```python
from build123d import *

# Parameters (mm, degrees)
F1_DEPTH = 20


with BuildPart() as f1:
    # F0 (on Top) → F1 (new body)
    with BuildSketch(Plane.XY):
        with BuildLine():
            Line((-12, 1.6), (-12, 0))
            Line((-12, 0), (0, 0))
            Line((0, 0), (0, 10))
            Line((0, 10), (-18, 10))
            Line((-18, 10), (-18, 8.4))
            ThreePointArc((-18, 8.4), (-10.814003, 7.009238), (-3.505098, 7.4))
            Line((-3.505098, 7.4), (-3.505098, 1.6))
            Line((-3.505098, 1.6), (-12, 1.6))
        make_face()
    extrude(amount=F1_DEPTH)


solid = f1.part
```
Geometry: final body of the model. Coordinates: model frame, mm. A direction names the side the tool comes from. Give positions to 0.01 mm unless a question says otherwise; leave off trailing zeros. Loops run counter-clockwise (first coordinate to the right, second up) from the corner with the lowest first, then second, coordinate; pieces in that order, holes last. Notation, with made-up numbers: (71.5, 42) -> (98.5, 42) arc R19 cw to (98.5, 57) -> close; hole circle Ø2 at (43.25, 87). An arc over 180 degrees is marked (long way). Return JSON: item names as keys, results as strings.
Item 1: Pin query (flat end, axial travel): P1, Ø1.5, axis at y = 3.5, z = 8.5, coming from the -X side; P2, Ø0.8, axis at y = 1, z = 5, coming from the -X side. Return the tip coordinate at first contact, or that it passes through.
Filled in:
{"P1": "x = -3.51", "P2": "x = -12"}
Item 2: Section D-D, the plane x = -7.25. Output: boundary loops of the cut face in (y, z), plus the area to 3 significant figures.
Filled in:
{"outline": "(0, 0) -> (1.6, 0) -> (1.6, 20) -> (0, 20) -> close; (6.98, 0) -> (10, 0) -> (10, 20) -> (6.98, 20) -> close", "area": "92.5 mm^2"}
Item 3: Section A-A, the plane z = 4. Output: boundary loops of the cut face in (x, y).
Filled in:
{"outline": "(-18, 8.4) arc R30 ccw to (-3.51, 7.4) -> (-3.51, 1.6) -> (-12, 1.6) -> (-12, 0) -> (0, 0) -> (0, 10) -> (-18, 10) -> close"}
Item 4: Section C-C, the plane y = 0.75. Output: boundary loops of the cut face in (x, z), plus the area to 3 significant figures.
Filled in:
{"outline": "(-12, 0) -> (0, 0) -> (0, 20) -> (-12, 20) -> close", "area": "240 mm^2"}
Item 5: Access query for faces 4 (the flat face through (-8, 1.6, 10)), 5 (the flat face through (-9, 10, 10)). Directions: +Z, -Z, +X, -X, +Y, -Y. A direction counts if a zero-diameter tool reaches every point of the face in a straight line with its end or side. Return the directions, or none.
Filled in:
{"face 4": "+Z, -Z, -X", "face 5": "+Z, -Z, +X, -X, +Y"}
Item 6: Mould query, pull axis X, two halves, no side actions, for faces 1 (the cylindrical face through (-10.916, 7.016, 9.86)), 2 (the flat face through (-7.1, 7.3, 0)), 3 (the flat face through (-12, 1, 10)). Classes: released by +X, released by -X, zero draft, split by the parting line, or undercut.
Filled in:
{"face 1": "undercut", "face 2": "zero draft", "face 3": "released by -X"}
Item 7: Section B-B, the plane x = -9.5. Output: boundary loops of the cut face in (y, z).
Filled in:
{"outline": "(0, 0) -> (1.6, 0) -> (1.6, 20) -> (0, 20) -> close; (6.95, 0) -> (10, 0) -> (10, 20) -> (6.95, 20) -> close"}
Item 8: Line query: line 1 (X direction, y = 6, z = 18.25); line 2 (Y direction, x = -14, z = 9.25); line 3 (Y direction, x = -4.25, z = 17.5). Output: solid intervals per line, ascending.
Filled in:
{"line 1": "-3.51 to 0", "line 2": "7.4 to 10", "line 3": "0 to 1.6, 7.28 to 10"}
